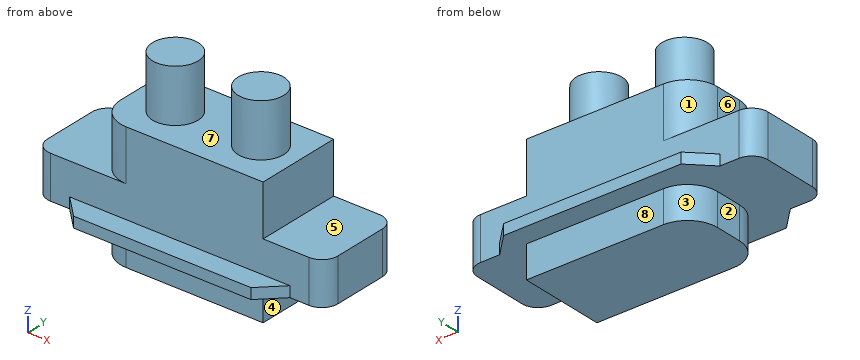
from build123d import *

# Parameters (mm, degrees)
DODANIE_WYCI_GNI_CIE1_DEPTH = 3
DODANIE_WYCI_GNI_CIE2_DEPTH = 1
SFAZOWANIE1_SIZE            = 2
DODANIE_WYCI_GNI_CIE3_DEPTH = 3
DODANIE_WYCI_GNI_CIE4_START = 7
DODANIE_WYCI_GNI_CIE4_DEPTH = 4.75
SZKIC6_R                    = 2.13
DODANIE_WYCI_GNI_CIE5_DEPTH = 4.95


with BuildPart() as part:
    # Szkic1 → Dodanie-wyciągnięcie1 (new body)
    with BuildSketch(Plane.XY):
        with BuildLine():
            Line((2.8, 0), (15.6, 0))
            Line((15.6, 0), (15.6, 8.1))
            Line((15.6, 8.1), (2.8, 8.1))
            ThreePointArc((2.8, 8.1), (0.820101013, 7.279898987), (0, 5.3))
            Line((0, 5.3), (0, 2.8))
            ThreePointArc((0, 2.8), (0.820101013, 0.820101013), (2.8, 0))
        make_face()
    extrude(amount=DODANIE_WYCI_GNI_CIE1_DEPTH)

    # Szkic2 → Dodanie-wyciągnięcie2 (add)
    with BuildSketch(Plane.XY.offset(3)):
        with BuildLine():
            Line((-0.49, 10.1), (16.1, 10.1))
            Line((16.1, 10.1), (16.1, 8.1))
            Line((16.1, 8.1), (19.88, 8.1))
            ThreePointArc((19.88, 8.1), (20.940660172, 7.660660172), (21.38, 6.6))
            Line((21.38, 6.6), (21.38, 1.5))
            ThreePointArc((21.38, 1.5), (20.940660172, 0.439339828), (19.88, 0))
            Line((19.88, 0), (16.1, 0))
            Line((16.1, 0), (16.1, -2))
            Line((16.1, -2), (-0.49, -2))
            Line((-0.49, -2), (-0.49, 0))
            Line((-0.49, 0), (-4.27, 0))
            ThreePointArc((-4.27, 0), (-5.330660172, 0.439339828), (-5.77, 1.5))
            Line((-5.77, 1.5), (-5.77, 6.6))
            ThreePointArc((-5.77, 6.6), (-5.330660172, 7.660660172), (-4.27, 8.1))
            Line((-4.27, 8.1), (-0.49, 8.1))
            Line((-0.49, 8.1), (-0.49, 10.1))
        make_face()
    extrude(amount=DODANIE_WYCI_GNI_CIE2_DEPTH)

    # Sfazowanie1
    sfazowanie1_edges = [part.edges().sort_by_distance(p)[0] for p in [
        (16.1, 8.1, 3.5),
        (16.1, 0, 3.5),
        (-0.49, 0, 3.5),
        (-0.49, 8.1, 3.5),
    ]]
    chamfer(sfazowanie1_edges, length=SFAZOWANIE1_SIZE - 0.0001)  # a hair under: the kernel refuses the full size

    # Szkic4 → Dodanie-wyciągnięcie3 (add)
    with BuildSketch(Plane.XY.offset(4)):
        with BuildLine():
            Line((19.88, 8.1), (18.1, 8.1))
            Line((18.1, 8.1), (-2.49, 8.1))
            Line((-2.49, 8.1), (-4.27, 8.1))
            ThreePointArc((-4.27, 8.1), (-5.330660172, 7.660660172), (-5.77, 6.6))
            Line((-5.77, 6.6), (-5.77, 1.5))
            ThreePointArc((-5.77, 1.5), (-5.330660172, 0.439339828), (-4.27, 0))
            Line((-4.27, 0), (-2.49, 0))
            Line((-2.49, 0), (18.1, 0))
            Line((18.1, 0), (19.88, 0))
            ThreePointArc((19.88, 0), (20.940660172, 0.439339828), (21.38, 1.5))
            Line((21.38, 1.5), (21.38, 6.6))
            ThreePointArc((21.38, 6.6), (20.940660172, 7.660660172), (19.88, 8.1))
        make_face()
    extrude(amount=DODANIE_WYCI_GNI_CIE3_DEPTH)

    # Szkic1<2> → Dodanie-wyciągnięcie4 (add)
    with BuildSketch(Plane.XY.offset(DODANIE_WYCI_GNI_CIE4_START)):
        with BuildLine():
            Line((2.8, 0), (15.6, 0))
            Line((15.6, 0), (15.6, 8.1))
            Line((15.6, 8.1), (2.8, 8.1))
            ThreePointArc((2.8, 8.1), (0.820101013, 7.279898987), (0, 5.3))
            Line((0, 5.3), (0, 2.8))
            ThreePointArc((0, 2.8), (0.820101013, 0.820101013), (2.8, 0))
        make_face()
    extrude(amount=DODANIE_WYCI_GNI_CIE4_DEPTH)

    # Szkic6 → Dodanie-wyciągnięcie5 (add)
    with BuildSketch(Plane.XY.offset(11.75)):
        with Locations(Location((4.1, 4.05, 0), (0, 0, 180))):
            Circle(SZKIC6_R)
        with Locations(Location((12.1, 4.05, 0), (0, 0, 180))):
            Circle(SZKIC6_R)
    extrude(amount=DODANIE_WYCI_GNI_CIE5_DEPTH)


solid = part.part
Geometry: final body of the model. Coordinates: model frame, mm. Face numbers are marked on the shaded views. A direction names the side the tool comes from. Coordinates: 2 decimals unless noted, no trailing zeros. Loops run counter-clockwise (first coordinate to the right, second up) from the corner with the lowest first, then second, coordinate; pieces in that order, holes last. Notation, with made-up numbers: M 8,0.5 L 66,0.5 A14 ccw 66,23.5 Z; hole C -27,65.5 d3. An arc over 180 degrees is marked long. One line per item, written item: value. Start each with the question number.
1) Reachability of the marked faces 1, 2, 3, 4 and 5 from +Z, -Z, +X, -X, +Y, -Y: full face, straight path, thin tool, end or side. Return the list, or none.
2) Cut plane C-C (y = 4.05). Return loops of the section in (x, z).
3) Material intervals for L1, parallel to Z at x = 19.75, y = 4; L2, parallel to Z at x = 8, y = 4; L3, parallel to Y at x = 14.5, z = 10, sorted ascending. Write a range as from..to.
4) Cut plane B-B (z = 15.5). Return loops of the section in (x, y), then the cut area to 3 significant figures.
5) Draft query along X for the marked faces 6, 7 and 8. Return one class per face: released by +X, released by -X, zero draft, split by the parting line, or undercut.
6) Cut plane A-A (x = 12.1). Return loops of the section in (y, z), then the cut area to 3 significant figures.
7) Pin query (flat end, axial travel): P1, Ø3, axis at y = 4.5, z = 10, coming from the -X side; P2, Ø2.5, axis at x = 6.5, z = 9, coming from the -Y side; P3, Ø2.5, axis at y = 4.5, z = 1, coming from the +X side. Return the tip coordinate at first contact, or that it passes through.
8) Cut plane D-D (z = 5.25). Return loops of the section in (x, y).
Evaluation:
1. face 1: +Z, -X, +Y
1. face 2: -Z, -X, +Y, -Y
1. face 3: -Z, -X, +Y
1. face 4: -Z, +X, +Y, -Y
1. face 5: +Z, +X, +Y, -Y
2. outline: M -5.77,3 L 0,3 L 0,0 L 15.6,0 L 15.6,3 L 21.38,3 L 21.38,7 L 15.6,7 L 15.6,11.75 L 14.23,11.75 L 14.23,16.7 L 9.97,16.7 L 9.97,11.75 L 6.23,11.75 L 6.23,16.7 L 1.97,16.7 L 1.97,11.75 L 0,11.75 L 0,7 L -5.77,7 Z
3. L1: 3..7
3. L2: 0..11.75
3. L3: 0..8.1
4. outline: C 4.1,4.05 d4.26; C 12.1,4.05 d4.26
4. area: 28.5 mm^2
5. face 6: released by -X
5. face 7: undercut
5. face 8: zero draft
6. outline: M -2,3 L 0,3 L 0,0 L 8.1,0 L 8.1,3 L 10.1,3 L 10.1,4 L 8.1,4 L 8.1,11.75 L 6.18,11.75 L 6.18,16.7 L 1.92,16.7 L 1.92,11.75 L 0,11.75 L 0,4 L -2,4 Z
6. area: 120 mm^2
7. P1: x = 0
7. P2: y = 0
7. P3: x = 15.6
8. outline: M -5.77,1.5 A1.5 ccw -4.27,0 L 19.88,0 A1.5 ccw 21.38,1.5 L 21.38,6.6 A1.5 ccw 19.88,8.1 L -4.27,8.1 A1.5 ccw -5.77,6.6 Z
